from build123d import *

# Parameters (mm, degrees)
SKETCH1_R               = 23.8125
SKETCH1_R_2             = 21.2725
BOSS_EXTRUDE1_DEPTH     = 27.94
SKETCH2_W               = 24.892
SKETCH2_H               = 1.27
SKETCH5_R               = 21.2725
BOSS_EXTRUDE2_DEPTH     = 0.635
CUT_EXTRUDE2_DEPTH      = 37.706625253
CUT_EXTRUDE2_DEPTH_BACK = 37.706625253
SKETCH7_R               = 5.08
BOSS_EXTRUDE7_DEPTH     = 15.875
SKETCH8_R               = 2.54
CUT_EXTRUDE3_DEPTH      = 19.05


with BuildPart() as part:
    # Sketch1 → Boss-Extrude1 (new body)
    with BuildSketch(Plane.XY):
        Circle(SKETCH1_R)
        Circle(SKETCH1_R_2, mode=Mode.SUBTRACT)
    extrude(amount=BOSS_EXTRUDE1_DEPTH)

    # Sketch2 → Cut-Revolve2 (revolve, cut)
    with BuildSketch(Plane(origin=(0, 0, 0), x_dir=(0, 0, -1), z_dir=(1, 0, 0))):
        with Locations((-13.97, 23.1775)):
            Rectangle(SKETCH2_W, SKETCH2_H)
    revolve(axis=Axis((0, 0, 0), (0, 0, 1)), mode=Mode.SUBTRACT)

    # Sketch5 → Boss-Extrude2 (add, symmetric)
    with BuildSketch(Plane.XY.offset(13.97)):
        Circle(SKETCH5_R)
    extrude(amount=BOSS_EXTRUDE2_DEPTH, both=True)

    # Sketch6 → Cut-Extrude2 (cut, two sides: drawn at the far end of the back side and taken through both)
    with BuildSketch(Plane.XY.offset(14.605).offset(-CUT_EXTRUDE2_DEPTH_BACK)):
        with BuildLine():
            Line((0, 5.08), (0, 20.076289255))
            ThreePointArc((0, 20.076289255), (6.203914564, 19.093685719), (11.800546745, 16.242059191))
            Line((11.800546745, 16.242059191), (2.985949082, 4.109806331))
            ThreePointArc((2.985949082, 4.109806331), (1.569806331, 4.831367103), (0, 5.08))
        make_face()
        with BuildLine():
            Line((4.831367103, 1.569806331), (19.093685719, 6.203914564))
            ThreePointArc((19.093685719, 6.203914564), (20.076289255, 0), (19.093685719, -6.203914564))
            Line((19.093685719, -6.203914564), (4.831367103, -1.569806331))
            ThreePointArc((4.831367103, -1.569806331), (5.08, 0), (4.831367103, 1.569806331))
        make_face()
        with BuildLine():
            Line((2.985949082, -4.109806331), (11.800546745, -16.242059191))
            ThreePointArc((11.800546745, -16.242059191), (6.203914564, -19.093685719), (0, -20.076289255))
            Line((0, -20.076289255), (0, -5.08))
            ThreePointArc((0, -5.08), (1.569806331, -4.831367103), (2.985949082, -4.109806331))
        make_face()
        with BuildLine():
            Line((-2.985949082, -4.109806331), (-11.800546745, -16.242059191))
            ThreePointArc((-11.800546745, -16.242059191), (-16.242059191, -11.800546745), (-19.093685719, -6.203914564))
            Line((-19.093685719, -6.203914564), (-4.831367103, -1.569806331))
            ThreePointArc((-4.831367103, -1.569806331), (-4.109806331, -2.985949082), (-2.985949082, -4.109806331))
        make_face()
        with BuildLine():
            Line((-4.831367103, 1.569806331), (-19.093685719, 6.203914564))
            ThreePointArc((-19.093685719, 6.203914564), (-16.242059191, 11.800546745), (-11.800546745, 16.242059191))
            Line((-11.800546745, 16.242059191), (-2.985949082, 4.109806331))
            ThreePointArc((-2.985949082, 4.109806331), (-4.109806331, 2.985949082), (-4.831367103, 1.569806331))
        make_face()
    extrude(amount=CUT_EXTRUDE2_DEPTH + CUT_EXTRUDE2_DEPTH_BACK, mode=Mode.SUBTRACT)

    # Sketch7 → Boss-Extrude7 (add)
    with BuildSketch(Plane.XY.offset(14.605)):
        Circle(SKETCH7_R)
    extrude(amount=BOSS_EXTRUDE7_DEPTH)

    # Sketch8 → Cut-Extrude3 (cut)
    with BuildSketch(Plane.XY.offset(30.48)):
        Circle(SKETCH8_R)
    extrude(amount=-CUT_EXTRUDE3_DEPTH, mode=Mode.SUBTRACT)


solid = part.part
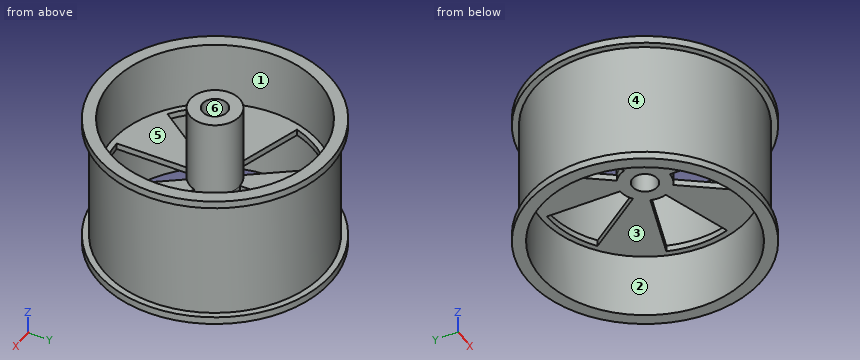
Verification items for the finished model (mm, model axes). Face numbers are marked on the shaded views. A direction names the side the tool comes from. Give positions to 0.01 mm unless a question says otherwise; leave off trailing zeros. Write each loop counter-clockwise with the first axis right and the second up, starting at its lowest first coordinate (ties: lowest second). Pieces come first, ordered by that corner, then holes.
(1) Mould release check, pull along Z, two halves, no side actions. Record for the marked faces 3, 4, 5 and 6: +Z half, -Z half, draft (parallel to the pull), parting line (faces both ways), or undercut.
(2) Cross-section at A-A (z = 19). Enter the section's corners in (x, y) (1 decimal), plus the area to 3 significant figures.
(3) Cross-section at B-B (y = 13). Enter the section's corners in (x, z) (3 decimals), plus the area to 3 significant figures.
(4) Access from +Z, -Z, +X, -X, +Y, -Y to the whole of each face (thin tool, end or side, straight path). Record for the marked faces 1 and 2.
(5) Gauge pin test, flat ends, axial feed: pin 1 (10 mm diameter, centred on y = -8.5, z = 14.5, fed in from -X); pin 2 (1 mm diameter, centred on x = 12.5, y = 8.5, fed in from -Z) (3 decimals); pin 3 (8 mm diameter, centred on x = 12, y = 1.5, fed in from +Z) (3 decimals); pin 4 (8 mm diameter, centred on x = 17.5, y = 15, fed in from -Z). Record the tip position at first contact, or that the pin passes through.
(6) Cross-section at D-D (y = 19). Enter the section's corners in (x, z) (3 decimals), plus the area to 3 significant figures.
(7) Material ranges on line 1 (Y direction, x = 0, z = 17.5); line 2 (X direction, y = -1.5, z = 13.5); line 3 (Y direction, x = -4.5, z = 26), recorded low to high.
(8) Cross-section at C-C (x = -6). Enter the section's corners in (y, z) (3 decimals), plus the area to 3 significant figures.
Worked out:
1. face 3: -Z half
1. face 4: undercut
1. face 5: +Z half
1. face 6: draft
2. outline: circle Ø45.1 at (0, 0); circle Ø10.2 at (0, 0); hole circle Ø42.5 at (0, 0); hole circle Ø5.1 at (0, 0)
2. area: 236 mm2
3. outline: (-19.951, 0) - (-16.838, 0) - (-16.838, 13.335) - (-15.299, 13.335) - (-15.299, 14.605) - (-16.838, 14.605) - (-16.838, 27.94) - (-19.951, 27.94) - (-19.951, 26.416) - (-18.416, 26.416) - (-18.416, 1.524) - (-19.951, 1.524) - close; (-9.445, 13.335) - (0, 13.335) - (0, 14.605) - (-9.445, 14.605) - close; (9.445, 13.335) - (16.838, 13.335) - (16.838, 0) - (19.951, 0) - (19.951, 1.524) - (18.416, 1.524) - (18.416, 26.416) - (19.951, 26.416) - (19.951, 27.94) - (16.838, 27.94) - (16.838, 14.605) - (9.445, 14.605) - close
3. area: 121 mm2
4. face 1: +Z
4. face 2: -Z
5. pin 1: stops at x = -22.27
5. pin 2: stops at z = 13.335
5. pin 3: stops at z = 14.605
5. pin 4: stops at z = 0
6. outline: (-14.354, 0) - (-9.567, 0) - (-9.567, 13.335) - (0, 13.335) - (0, 14.605) - (-9.567, 14.605) - (-9.567, 27.94) - (-14.354, 27.94) - (-14.354, 26.416) - (-12.131, 26.416) - (-12.131, 1.524) - (-14.354, 1.524) - close; (6.485, 13.335) - (9.567, 13.335) - (9.567, 0) - (14.354, 0) - (14.354, 1.524) - (12.131, 1.524) - (12.131, 26.416) - (14.354, 26.416) - (14.354, 27.94) - (9.567, 27.94) - (9.567, 14.605) - (6.485, 14.605) - close
6. area: 173 mm2
7. line 1: y = -22.54 to -21.27, -5.08 to -2.54, 2.54 to 5.08, 21.27 to 22.54
7. line 2: x = -22.49 to -2.05, 2.05 to 4.85, 20.02 to 22.49
7. line 3: y = -22.09 to -20.79, -2.36 to 2.36, 20.79 to 22.09
8. outline: (-23.044, 0) - (-20.409, 0) - (-20.409, 13.335) - (-8.258, 13.335) - (-8.258, 14.605) - (-20.409, 14.605) - (-20.409, 27.94) - (-23.044, 27.94) - (-23.044, 26.416) - (-21.729, 26.416) - (-21.729, 1.524) - (-23.044, 1.524) - close; (-1.95, 13.335) - (1.95, 13.335) - (1.95, 14.605) - (-1.95, 14.605) - close; (8.258, 13.335) - (20.409, 13.335) - (20.409, 0) - (23.044, 0) - (23.044, 1.524) - (21.729, 1.524) - (21.729, 26.416) - (23.044, 26.416) - (23.044, 27.94) - (20.409, 27.94) - (20.409, 14.605) - (8.258, 14.605) - close
8. area: 118 mm2
